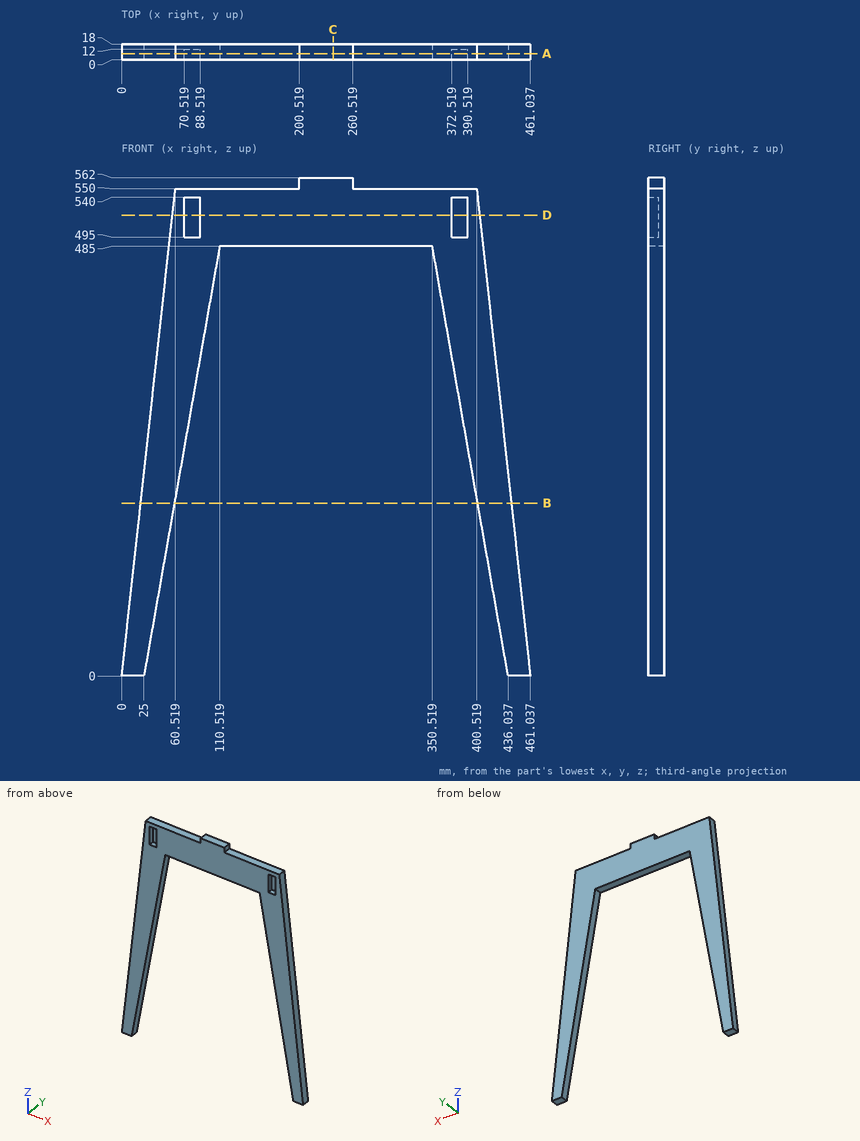
Check sheet for the drawn part. Datum: minimum x, y, z corner. Units: mm. Coordinates: 2 decimals unless noted, no trailing zeros. Loops run counter-clockwise (first coordinate to the right, second up) from the corner with the lowest first, then second, coordinate; pieces in that order, holes last. Notation, with made-up numbers: (32.25, -12) -> (71.25, -12) arc R31 cw to (71.25, 22) -> close; hole circle Ø6 at (67, 80.5). An arc over 180 degrees is marked (long way). Answer as a JSON object with one key per item and string values. Group by question number.
Item 1: Scan lines: probe 1 along Z at (x, y) = (291, 1); probe 2 along Z at (x, y) = (256, 4.5); probe 3 along X at (y, z) = (5, 55) (1 decimal). Record each from-to range of solid material in increasing order.
Item 2: Sectioned sample at D-D on z = 520. Record the boundary of the cut face in (x, y), plus the area to 3 significant figures.
Item 3: Depth check by flat-ended pin: pin 1 (4 mm diameter, centred on y = 15.5, z = 57.5, fed in from +X); pin 2 (5.5 mm diameter, centred on x = 356, y = 8, fed in from +Z); pin 3 (9.5 mm diameter, centred on y = 10.5, z = 553.5, fed in from +X). Enter the tip coordinate at first touch or a pass-through.
Item 4: Sectioned sample at C-C on x = 238.5. Record the boundary of the cut face in (y, z), plus the area to 3 significant figures.
Item 5: Sectioned sample at A-A on y = 7. Record the boundary of the cut face in (x, z), plus the area to 3 significant figures.
Item 6: Sectioned sample at B-B on z = 195. Record the boundary of the cut face in (x, y), plus the area to 3 significant figures.
Evaluation:
{
 "1": {"probe 1": "z = 485 to 550", "probe 2": "z = 485 to 562", "probe 3": "x = 6.1 to 34.7, 426.3 to 455"},
 "2": {"outline": "(57.22, 0) -> (70.52, 0) -> (70.52, 12) -> (88.52, 12) -> (88.52, 0) -> (372.52, 0) -> (372.52, 12) -> (390.52, 12) -> (390.52, 0) -> (403.82, 0) -> (403.82, 18) -> (57.22, 18) -> close", "area": "5,810 mm²"},
 "3": {"pin 1": "stops at x = 454.93", "pin 2": "stops at z = 550", "pin 3": "stops at x = 400.66"},
 "4": {"outline": "(0, 485) -> (18, 485) -> (18, 562) -> (0, 562) -> close", "area": "1,390 mm²"},
 "5": {"outline": "(0, 0) -> (25, 0) -> (110.52, 485) -> (350.52, 485) -> (436.04, 0) -> (461.04, 0) -> (400.52, 550) -> (260.52, 550) -> (260.52, 562) -> (200.52, 562) -> (200.52, 550) -> (60.52, 550) -> close; hole (70.52, 495) -> (88.52, 495) -> (88.52, 540) -> (70.52, 540) -> close; hole (372.52, 495) -> (390.52, 495) -> (390.52, 540) -> (372.52, 540) -> close", "area": "61,500 mm²"},
 "6": {"outline": "(21.46, 0) -> (59.38, 0) -> (59.38, 18) -> (21.46, 18) -> close; (401.65, 0) -> (439.58, 0) -> (439.58, 18) -> (401.65, 18) -> close", "area": "1,370 mm²"}
}
